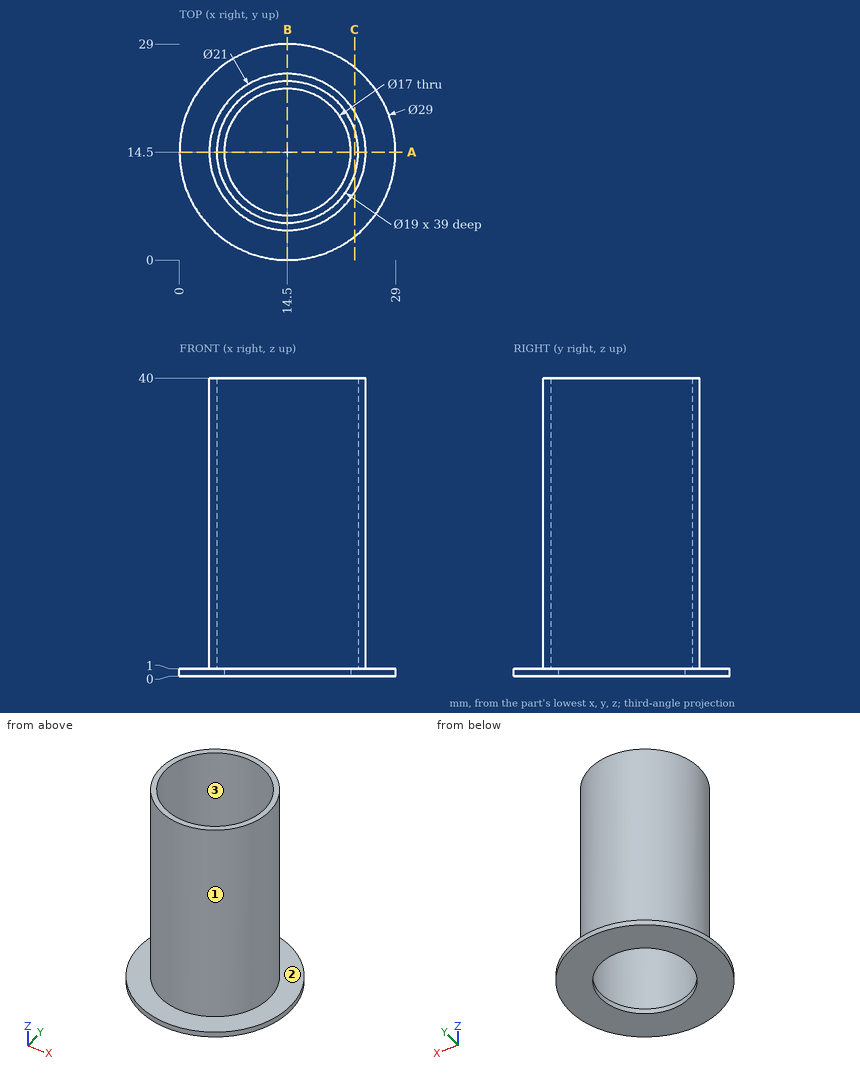
Verification items for this drawing (mm, ordinates from the low corner). Coordinates: 2 decimals unless noted, no trailing zeros. Write each loop counter-clockwise with the first axis right and the second up, starting at its lowest first coordinate (ties: lowest second). Pieces come first, ordered by that corner, then holes. Notation, with made-up numbers: M 51.25,9 L 95.25,9 A11 ccw 95.25,16 Z; hole C 82.5,53.25 d8. An arc over 180 degrees is marked long. One line per item, written item: value. Start each with the question number.
(1) Depth check by flat-ended pin: pin 1 (1 mm diameter, centred on x = 24.5, y = 22.5, fed in from -Z); pin 2 (5 mm diameter, centred on y = 22, z = 24.5, fed in from -X); pin 3 (12 mm diameter, centred on y = 13, z = 21, fed in from -X); pin 4 (9.5 mm diameter, centred on x = 12, y = 13, fed in from +Z). Enter the tip coordinate at first touch or a pass-through.
(2) Sectioned sample at C-C, the plane x = 23.5. Enter the section's corners in (y, z), and give its area (3 significant figures).
(3) Release check for a two-part mould opening along X. For the marked faces 1, 2 and 3 record: released by +X, released by -X, zero draft, split by the parting line, or undercut.
(4) Sectioned sample at A-A, the plane y = 14.5. Enter the section's corners in (x, z).
(5) Scan lines: line 1 along X through (y, z) = (14.5, 17.5); line 2 along Y through (x, z) = (14.5, 0.4). Record each from-to range of solid material in increasing order. Write a range as [from, to].
Filled sheet:
1. pin 1: z = 0
1. pin 2: x = 5.27
1. pin 3: x = 4
1. pin 4: through
2. outline: M 3.13,0 L 25.87,0 L 25.87,1 L 19.91,1 L 19.91,40 L 17.54,40 L 17.54,1 L 11.46,1 L 11.46,40 L 9.09,40 L 9.09,1 L 3.13,1 Z
2. area: 207 mm²
3. face 1: split by the parting line
3. face 2: zero draft
3. face 3: undercut
4. outline: M 0,0 L 6,0 L 6,1 L 5,1 L 5,40 L 4,40 L 4,1 L 0,1 Z; M 23,0 L 29,0 L 29,1 L 25,1 L 25,40 L 24,40 L 24,1 L 23,1 Z
5. line 1: [4, 5], [24, 25]
5. line 2: [0, 6], [23, 29]
